Check sheet for the modelled part. Datum: model origin and axes. Units: mm. Face numbers are marked on the shaded views. Coordinates: 2 decimals unless noted, no trailing zeros. Loops run counter-clockwise (first coordinate to the right, second up) from the corner with the lowest first, then second, coordinate; pieces in that order, holes last.
```python
from build123d import *

# Parameters (mm, degrees)
SKETCH1_W             = 139.954
SKETCH1_H             = 71.882
SKETCH1_R             = 4.191
BOSS_EXTRUDE1_DEPTH   = 3.175
SKETCH2_R             = 3.175
BOSS_EXTRUDE4_DEPTH   = 12.7
BOSS_EXTRUDE4_2_DEPTH = 12.7
SKETCH1_7_R           = 4.191
BOSS_EXTRUDE5_DEPTH   = 3.175
BOSS_EXTRUDE6_START   = -3.175
SKETCH14_R            = 4.191
BOSS_EXTRUDE6_DEPTH   = 3.175
SKETCH15_W            = 71.882
SKETCH15_H            = 3.175
CUT_EXTRUDE1_DEPTH    = 2.794
SKETCH16_W            = 71.882
SKETCH16_H            = 3.175
BOSS_EXTRUDE7_DEPTH   = 2.794


with BuildPart() as part:
    # Sketch1 → Boss-Extrude1 (new body)
    with BuildSketch(Plane(origin=(0, 0, 0), x_dir=(1, 0, 0), z_dir=(0, 1, 0))):
        with Locations((69.977, 35.941)):
            Rectangle(SKETCH1_W, SKETCH1_H)
        with Locations(Location((6.35, 35.941, 0), (0, 0, 270))):
            Circle(SKETCH1_R, mode=Mode.SUBTRACT)
        with Locations(Location((129.286, 35.941, 0), (0, 0, 270))):
            Circle(SKETCH1_R, mode=Mode.SUBTRACT)
    extrude(amount=-BOSS_EXTRUDE1_DEPTH)



with BuildPart() as body_2:
    # Sketch2 → Boss-Extrude4 (new body)
    with BuildSketch(Plane.XZ.offset(3.175)):
        with Locations(Location((6.35, -35.941, 0), (0, 0, 270))):
            Circle(SKETCH2_R)
    extrude(amount=-BOSS_EXTRUDE4_DEPTH)


with BuildPart() as body_3:
    # Sketch2 → Boss-Extrude4 2 (new body)
    with BuildSketch(Plane.XZ.offset(3.175)):
        with Locations(Location((129.286, -35.941, 0), (0, 0, 270))):
            Circle(SKETCH2_R)
    extrude(amount=-BOSS_EXTRUDE4_2_DEPTH)


with BuildPart() as part_1:
    add(part.part)

    add(body_3.part)  # Boss-Extrude5 merges body 3
    # Sketch1_7 → Boss-Extrude5 (add)
    with BuildSketch(Plane(origin=(0, 0, 0), x_dir=(1, 0, 0), z_dir=(0, 1, 0))):
        with Locations((129.286, 35.941)):
            Circle(SKETCH1_7_R)
    extrude(amount=-BOSS_EXTRUDE5_DEPTH)


    add(body_2.part)  # Boss-Extrude6 merges body 2
    # Sketch14 → Boss-Extrude6 (add)
    with BuildSketch(Plane.XZ.offset(3.175).offset(BOSS_EXTRUDE6_START)):
        with Locations((6.35, -35.941)):
            Circle(SKETCH14_R)
    extrude(amount=BOSS_EXTRUDE6_DEPTH)

    # Sketch15 → Cut-Extrude1 (cut)
    with BuildSketch(Plane.ZY):
        with Locations((-35.941, -1.5875)):
            Rectangle(SKETCH15_W, SKETCH15_H)
    extrude(amount=-CUT_EXTRUDE1_DEPTH, mode=Mode.SUBTRACT)

    # Sketch16 → Boss-Extrude7 (add)
    with BuildSketch(Plane(origin=(139.954, 0, 0), x_dir=(0, 0, -1), z_dir=(1, 0, 0))):
        with Locations((35.941, -1.5875)):
            Rectangle(SKETCH16_W, SKETCH16_H)
    extrude(amount=BOSS_EXTRUDE7_DEPTH)


solid = part_1.part
```
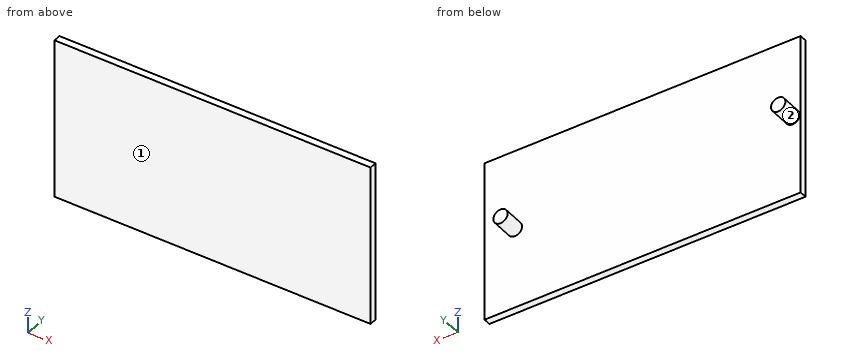
1) Section check A-A on x = 6.35. Enter the section's corners in (y, z) (3 decimals), plus the area to 3 significant figures.
Answer sheet:
outline: (-3.175, -71.882) - (0, -71.882) - (0, -39.116) - (9.525, -39.116) - (9.525, -32.766) - (0, -32.766) - (0, 0) - (-3.175, 0) - close
area: 289 mm2
2) Mould release check, pull along X, two halves, no side actions. Record for the marked faces 1 and 2: +X half, -X half, draft (parallel to the pull), parting line (faces both ways), or undercut.
Answer sheet:
face 1: draft
face 2: undercut
3) Depth check by flat-ended pin: pin 1 (3 mm diameter, centred on x = 51.5, z = -38.5, fed in from +Y). Enter the tip coordinate at first touch or a pass-through.
Answer sheet:
pin 1: stops at y = 0
4) Section check D-D on x = 86. Enter the section's corners in (y, z) (3 decimals), plus the area to 3 significant figures.
Answer sheet:
outline: (-3.175, -71.882) - (0, -71.882) - (0, 0) - (-3.175, 0) - close
area: 228 mm2
5) Section check B-B on z = -11. Enter the section's corners in (x, y) (3 decimals), plus the area to 3 significant figures.
Answer sheet:
outline: (2.794, -3.175) - (142.748, -3.175) - (142.748, 0) - (2.794, 0) - close
area: 444 mm2
6) Scan lines: line 1 (X direction, y = 5.5, z = -35.5); line 2 (Y direction, x = 106, z = -63.5) (3 decimals). Record each from-to range of solid material in increasing order.
Answer sheet:
line 1: x = 3.21 to 9.49, 126.14 to 132.43
line 2: y = -3.175 to 0
7) Section check C-C on y = 7.75. Enter the section's corners in (x, z) (3 decimals).
Answer sheet:
outline: circle Ø6.35 at (6.35, -35.941); circle Ø6.35 at (129.286, -35.941)
